For this review, take the finished solid that the model builds, in its own axes (mm). A direction names the side the tool comes from. Round coordinates to 2 decimals unless told otherwise and drop trailing zeros. Loops run counter-clockwise (first coordinate to the right, second up) from the corner with the lowest first, then second, coordinate; pieces in that order, holes last.
1) Wall thickness on L1, parallel to Y at x = 9.5, z = 6.75; L2, parallel to Y at x = 60.5, z = 1.9; L3, parallel to Y at x = 9.5, z = 3.75: over which ranges is each line inside the solid? List them lowest first.
2) Mouldability with a two-part tool opening along Y and no side actions: class faces 1 (the flat face through (22, 20, 3)), 2 (the flat face through (59, 10.12, 2)), 3 (the cylindrical face through (49.71, -16.76, 4.44)), 4 (the flat face through (51.3, -17.3, 9)) as pulls with the +Y half, pulls with the -Y half, needs draft (parallel to the pull), parting line crosses it, or undercut.
3) Take a section at B-B (x = 50.7). State the section outline as (y, z) points, then the cut area to 3 significant figures.
4) Take a section at C-C (z = 19). State the section outline as (x, y) points.
5) Take a section at A-A (z = 6). Give the number of separate pieces and of enclosed holes in the cut face, then the cut area to 3 significant figures.
6) Take a section at D-D (x = 60.5). State the section outline as (y, z) points.
7) Insertion check: pin 1 (4 mm diameter, centred on y = -10.5, z = 12, fed in from +X); pin 2 (1 mm diameter, centred on x = 1, z = 13.5, fed in from -Y); pin 3 (20 mm diameter, centred on x = 43.5, y = -4, fed in from +Z). Each pin has a flat end and moves straight along its axis. Give the tip position at first contact, or say it passes through.
8) Tool access review of faces 5 (the cylindrical face through (48.49, -13.97, 6.46)), 6 (the flat face through (2, -20, 12)), 7 (the flat face through (11, 16, 9)): name each direction out of +Z, -Z, +X, -X, +Y, -Y from which nothing blocks a thin tool from reaching the whole face with its end or side.
```python
from build123d import *

# Parameters (mm, degrees)
F0_R     = 3
F0_R_2   = 2.45
F1_DEPTH = 4
F0_R_3   = 1.25
F2_DEPTH = 9
F0_W     = 3.5
F0_H     = 40
F3_DEPTH = 25
F4_R     = 2.5
F5_DEPTH = 25


with BuildPart() as f1:
    # F0 (on Top) → F1 (new body)
    with BuildSketch(Plane.XY):
        with BuildLine():
            Line((54.6, 20), (3.5, 20))
            Line((3.5, 20), (3.5, -20))
            Line((3.5, -20), (3.5, -20.100027))
            Line((3.5, -20.100027), (55.5, -20.100027))
            Line((55.5, -20.100027), (55.5, 10.120172))
            Line((55.5, 10.120172), (62.5, 10.120172))
            ThreePointArc((62.5, 10.120172), (66.136013, 15.060086), (62.5, 20))
            Line((62.5, 20), (54.6, 20))
        make_face()
        with Locations((9.5, -16.000027)):
            Circle(F0_R, mode=Mode.SUBTRACT)
        with Locations((50.7, -16.000027)):
            Circle(F0_R, mode=Mode.SUBTRACT)
        with Locations((9.5, 15.9)):
            Circle(F0_R, mode=Mode.SUBTRACT)
        with Locations((50.7, 15.9)):
            Circle(F0_R, mode=Mode.SUBTRACT)
        with Locations((60.5, 15)):
            Circle(F0_R_2, mode=Mode.SUBTRACT)
    extrude(amount=F1_DEPTH)

    # F0 (on Top) → F2 (join)
    with BuildSketch(Plane.XY):
        with Locations((9.5, 15.9)):
            Circle(F0_R)
        with Locations((9.5, 15.9)):
            Circle(F0_R_3, mode=Mode.SUBTRACT)
        with Locations((50.7, 15.9)):
            Circle(F0_R)
        with Locations((50.7, 15.9)):
            Circle(F0_R_3, mode=Mode.SUBTRACT)
        with Locations((50.7, -16.000027)):
            Circle(F0_R)
        with Locations((50.7, -16.000027)):
            Circle(F0_R_3, mode=Mode.SUBTRACT)
        with Locations((9.5, -16.000027)):
            Circle(F0_R)
        with Locations((9.5, -16.000027)):
            Circle(F0_R_3, mode=Mode.SUBTRACT)
    extrude(amount=F2_DEPTH)

    # F0 (on Top) → F3 (join)
    with BuildSketch(Plane.XY):
        with Locations((1.75, 0)):
            Rectangle(F0_W, F0_H)
    extrude(amount=F3_DEPTH)

    # F4 (on Right) → F5 (cut)
    with BuildSketch(Plane.YZ):
        with Locations((13, 19)):
            Circle(F4_R)
        with Locations((-13, 19)):
            Circle(F4_R)
    extrude(amount=F5_DEPTH, mode=Mode.SUBTRACT)


solid = f1.part
```
Response:
1. L1: y = -19 to -17.25, -14.75 to -13, 12.9 to 14.65, 17.15 to 18.9
1. L2: y = 10.12 to 12.55, 17.45 to 20
1. L3: y = -20.1 to -17.25, -14.75 to 14.65, 17.15 to 20
2. face 1: pulls with the +Y half
2. face 2: pulls with the -Y half
2. face 3: undercut
2. face 4: needs draft
3. outline: (-20.1, 0) - (-17.25, 0) - (-17.25, 9) - (-19, 9) - (-19, 4) - (-20.1, 4) - close; (-14.75, 0) - (14.65, 0) - (14.65, 9) - (12.9, 9) - (12.9, 4) - (-13, 4) - (-13, 9) - (-14.75, 9) - close; (17.15, 0) - (20, 0) - (20, 4) - (18.9, 4) - (18.9, 9) - (17.15, 9) - close
3. area: 175 mm2
4. outline: (0, -20) - (3.5, -20) - (3.5, -15.5) - (0, -15.5) - close; (0, -10.5) - (3.5, -10.5) - (3.5, 10.5) - (0, 10.5) - close; (0, 15.5) - (3.5, 15.5) - (3.5, 20) - (0, 20) - close
5. separate pieces: 5
5. enclosed holes: 4
5. area: 233 mm2
6. outline: (10.12, 0) - (12.55, 0) - (12.55, 4) - (10.12, 4) - close; (17.45, 0) - (20, 0) - (20, 4) - (17.45, 4) - close
7. pin 1: stops at x = 3.5
7. pin 2: stops at y = -20
7. pin 3: stops at z = 4
8. face 5: +Z
8. face 6: +Z, -Z, -X, -Y
8. face 7: +Z, +X, +Y, -Y
